Work out the finished part from the listing and answer in its coordinate system (mm). Face numbers are marked on the shaded views. A direction names the side the tool comes from. Round coordinates to 2 decimals unless told otherwise and drop trailing zeros. Write each loop counter-clockwise with the first axis right and the second up, starting at its lowest first coordinate (ties: lowest second). Pieces come first, ordered by that corner, then holes. Notation, with made-up numbers: M 72.5,37 L 117.5,37 A18 cw 117.5,54 Z; hole C -31,37.25 d11. An arc over 180 degrees is marked long. Answer in a Markdown table with one row per item.
Autodesk Inventor part; units mm, degrees
ref_plane "YZ Plane" through (0, 0, 0) normal (1, 0, 0) x (0, 1, 0)
ref_plane "XZ Plane" through (0, 0, 0) normal (0, 1, 0) x (-1, 0, 0)
ref_plane "XY Plane" through (0, 0, 0) normal (0, 0, 1) x (1, 0, 0)
sketch "Szkic1" plane through (0, 0, 0) normal (0, 0, 1) x (1, 0, 0)
  line L0 (-12.5, -17.5) -> (12.5, -17.5)
  line L1 (12.5, -17.5) -> (12.5, 17.5)
  line L2 (12.5, 17.5) -> (-12.5, 17.5)
  line L3 (-12.5, 17.5) -> (-12.5, -17.5)
  line L4 (-12.5, -17.5) -> (12.5, 17.5) construction
  line L5 (12.5, -17.5) -> (-12.5, 17.5) construction
  line L6 (7.5, -12.5) -> (-7.5, -12.5) construction
  line L7 (-7.5, -12.5) -> (-7.5, 12.5) construction
  line L8 (-7.5, 12.5) -> (7.5, 12.5) construction
  line L9 (7.5, 12.5) -> (7.5, -12.5) construction
  line L10 (7.5, -12.5) -> (-7.5, 12.5) construction
  line L11 (-7.5, -12.5) -> (7.5, 12.5) construction
  point P0 (0, 0)
  dimension "d0" = 25
  dimension "d1" = 35
  dimension "d2" = 15
  dimension "d3" = 25
extrude "Wyciągnięcie proste1" add sketch "Szkic1" along normal blind 12
hole "Otwór1" at (-7.5, 12.5, 0) at (7.5, 12.5, 0) at (7.5, -12.5, 0) at (-7.5, -12.5, 0) direction (0, 0, 1) diameter 3.5 end through all
sketch "Szkic2" plane through (-12.5, 17.5, 0) normal (0, 1, 0) x (1, 0, 0)
  line L0 (25, -12) -> (0, -12)
  line L1 (12.5, 0) -> (12.5, -12) construction
  line L2 (8.4, -12) -> (8.4, -8.5)
  arc A0 (16.6, -8.5) -> (8.4, -8.5) centre (12.5, -8.5) ccw
  line L3 (16.6, -8.5) -> (16.6, -12)
  dimension "d13" = 4.1
  dimension "d15" = 3.5
extrude "Wyciągnięcie proste2" cut sketch "Szkic2" against normal blind 28
properties part number "roll_mount2"
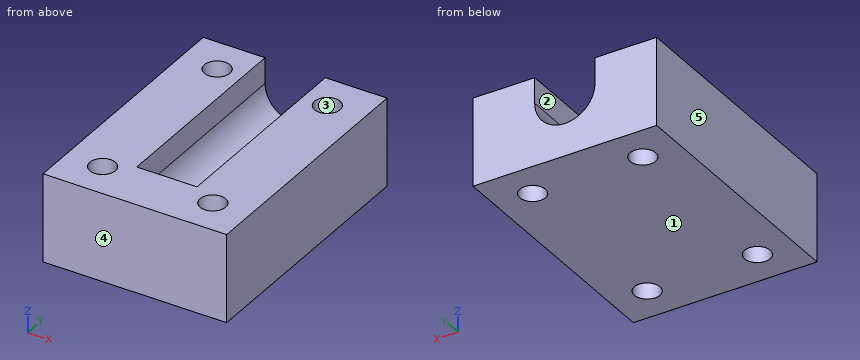
1. Given pin 1 (2 mm diameter, centred on x = 2, z = 8, fed in from +Y), flat-ended and moving along its own axis, determine where the tip first touches the part or whether it passes through.
Calculated:
| item | result |
|---|---|
| pin 1 | stops at y = -10.5 |
2. A tool of negligible diameter and unlimited length cuts with its end or side. For the marked faces 1 and 2, from which of +Z, -Z, +X, -X, +Y, -Y can it reach the whole face along a straight path? Write none if from no direction.
Calculated:
| item | result |
|---|---|
| face 1 | -Z, +X, -X, +Y, -Y |
| face 2 | +Z, +Y |
3. Determine the mould class of the marked faces 3, 4 and 5 for opening direction X: released by +X, released by -X, zero draft, split by the parting line, or undercut.
Calculated:
| item | result |
|---|---|
| face 3 | undercut |
| face 4 | zero draft |
| face 5 | released by -X |
4. Consider line 1 along X through (y, z) = (-12.5, 8.5); line 2 along Y through (x, z) = (-7.5, 3.5); line 3 along X through (y, z) = (8, 9.75). Determine where each line is inside the solid, lowest interval first. Write a range as from..to.
Calculated:
| item | result |
|---|---|
| line 1 | x = -12.5..-9.25, -5.75..5.75, 9.25..12.5 |
| line 2 | y = -17.5..-14.25, -10.75..10.75, 14.25..17.5 |
| line 3 | x = -12.5..-4.1, 4.1..12.5 |
5. The part is cut by section D-D (y = 4). Determine the outline of the cut face in (x, z), plus the area to 3 significant figures.
Calculated:
| item | result |
|---|---|
| outline | M -12.5,0 L 12.5,0 L 12.5,12 L 4.1,12 L 4.1,8.5 A4.1 cw -4.1,8.5 L -4.1,12 L -12.5,12 Z |
| area | 245 mm² |
6. The part is cut by section B-B (x = 7.5). Determine the outline of the cut face in (y, z), plus the area to 3 significant figures.
Calculated:
| item | result |
|---|---|
| outline | M -17.5,0 L -14.25,0 L -14.25,12 L -17.5,12 Z; M -10.75,0 L 10.75,0 L 10.75,12 L -10.75,12 Z; M 14.25,0 L 17.5,0 L 17.5,12 L 14.25,12 Z |
| area | 336 mm² |
7. The part is cut by section A-A (y = -12.5). Determine the outline of the cut face in (x, z), plus the area to 3 significant figures.
Calculated:
| item | result |
|---|---|
| outline | M -12.5,0 L -9.25,0 L -9.25,12 L -12.5,12 Z; M -5.75,0 L 5.75,0 L 5.75,12 L -5.75,12 Z; M 9.25,0 L 12.5,0 L 12.5,12 L 9.25,12 Z |
| area | 216 mm² |
8. The part is cut by section C-C (z = 7.25). Determine the outline of the cut face in (x, y), plus the area to 3 significant figures.
Calculated:
| item | result |
|---|---|
| outline | M -12.5,-17.5 L 12.5,-17.5 L 12.5,17.5 L 3.9,17.5 L 3.9,-10.5 L -3.9,-10.5 L -3.9,17.5 L -12.5,17.5 Z; hole C -7.5,-12.5 d3.5; hole C -7.5,12.5 d3.5; hole C 7.5,-12.5 d3.5; hole C 7.5,12.5 d3.5 |
| area | 618 mm² |
